from build123d import *

# Parameters (mm, degrees)
F0_W           = 129.3
F0_H           = 64.2
F1_DEPTH       = 50.5
F3_D           = 16
F3_DEPTH       = 16
F3_CBORE_D     = 44
F3_CBORE_DEPTH = 16
F3_TIP         = 4.8068849522


with BuildPart() as f1:
    # F0 (on Front) → F1 (new body)
    with BuildSketch(Plane.XZ):
        with Locations((-31.8797686338, 21.3420945689)):
            Rectangle(F0_W, F0_H)
    extrude(amount=F1_DEPTH)

    # F3
    with Locations(Plane.XZ.offset(50.5)):
        with Locations((-52.0297686338, 21.3420945689)):
            CounterBoreHole(F3_D / 2, F3_CBORE_D / 2, F3_CBORE_DEPTH, depth=F3_DEPTH)
            with Locations((0, 0, -(F3_DEPTH + F3_TIP / 2))):  # 118° drill point
                Cone(0, F3_D / 2, F3_TIP, mode=Mode.SUBTRACT)


solid = f1.part
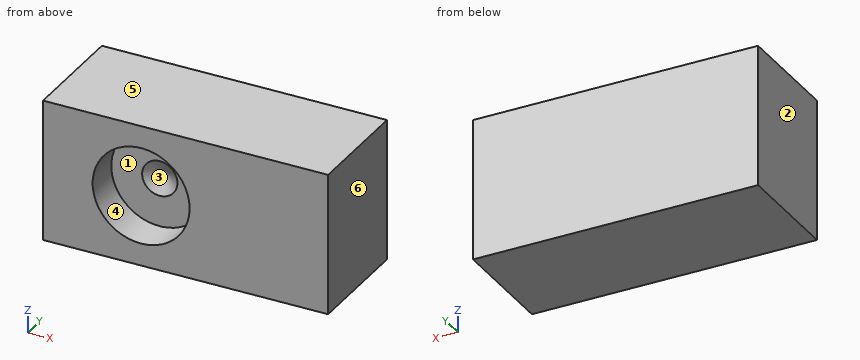
Source: CAD feature listing. Evaluate the final solid. Frame: model axes, mm. Face numbers are marked on the shaded views. A direction names the side the tool comes from. Coordinates: 2 decimals unless noted, no trailing zeros. Order: outer loops, then holes, each group sorted by start corner. A loop starts at its lowest first (then second) coordinate and runs counter-clockwise, first axis right, second up. Notation, with made-up numbers: M 66.5,-4 L 71.5,-4 A20 cw 71.5,26 Z; hole C -2.5,-1 d4. An arc over 180 degrees is marked long. Write each question's results on one line, items separated by ' | '. Start each with the question number.
Item 1: First-contact query: pin 1 Ø22 at (x, z) = (-61.5, 18) entering from -Y. Flat tip, straight axial feed; report the tip coordinate or a pass-through.
Item 2: Draft query along X for the marked faces 3, 4, 5 and 6. Return one class per face: pulls with the +X half, pulls with the -X half, needs draft (parallel to the pull), parting line crosses it, or undercut.
Item 3: Set-up query: the marked faces 1 and 2. Return all of +Z, -Z, +X, -X, +Y, -Y with unobstructed straight access to the full face (end or side cutting, diameter ignored); none if empty.
Item 4: Line query: probe 1 along X at (y, z) = (-42, 6.5); probe 2 along Y at (x, z) = (-50.5, 11); probe 3 along X at (y, z) = (-42, 36.5). Output: solid intervals per line, ascending.
Item 5: Cut plane A-A (y = -43.5). Return loops of the section in (x, z), and give its area (3 significant figures).
Item 6: Cut plane C-C (x = -31.5). Return loops of the section in (y, z).
Item 7: Cut plane B-B (z = 11). Return loops of the section in (x, y), and give its area (3 significant figures).
Checked values:
1) pin 1: stops at y = -34.5
2) face 3: undercut | face 4: undercut | face 5: needs draft | face 6: pulls with the +X half
3) face 1: -Y | face 2: +Z, -Z, -X, +Y, -Y
4) probe 1: x = -96.53 to -68.27, -35.79 to 32.77 | probe 2: y = -34.5 to 0 | probe 3: x = -96.53 to -67.97, -36.08 to 32.77
5) outline: M -96.53,-10.76 L 32.77,-10.76 L 32.77,53.44 L -96.53,53.44 Z; hole C -52.03,21.34 d44 | area: 6,780 mm2
6) outline: M -50.5,-10.76 L 0,-10.76 L 0,53.44 L -50.5,53.44 L -50.5,29.25 L -34.5,29.25 L -34.5,13.43 L -50.5,13.43 Z
7) outline: M -96.53,-50.5 L -71.45,-50.5 L -71.45,-34.5 L -32.61,-34.5 L -32.61,-50.5 L 32.77,-50.5 L 32.77,0 L -96.53,0 Z | area: 5,910 mm2
